Geometry: final body of the model. Coordinates: model frame, mm. Coordinates: 2 decimals unless noted, no trailing zeros. Order: outer loops, then holes, each group sorted by start corner. A loop starts at its lowest first (then second) coordinate and runs counter-clockwise, first axis right, second up. Notation, with made-up numbers: M 26,80 L 58,80 A31 cw 58,115 Z; hole C 88.25,-30 d10. An arc over 180 degrees is marked long. Write item = value, one per line. Start each with the question number.
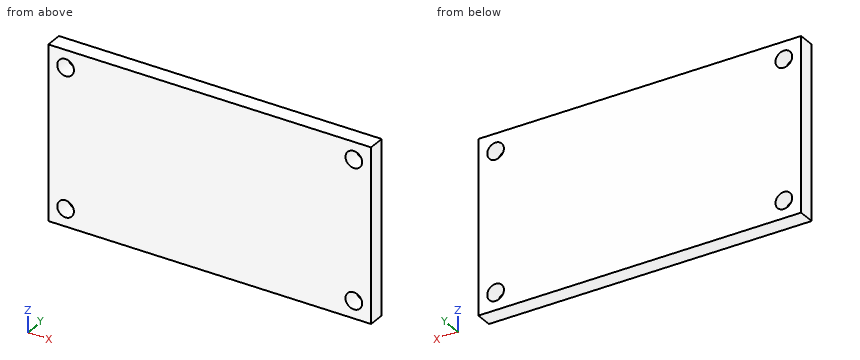
```python
from build123d import *

# Parameters (mm, degrees)
SKETCH1_W               = 58
SKETCH1_H               = 31
BOSS_EXTRUDE1_DEPTH     = 3
SKETCH2_R               = 1.5
CUT_EXTRUDE1_DEPTH      = 34.018933962
MIRROR2_COPY_1_SKETCH_R = 1.5
MIRROR2_COPY_1_DEPTH    = 34.018933962


with BuildPart() as part:
    # Sketch1 → Boss-Extrude1 (new body)
    with BuildSketch(Plane(origin=(0, 0, 0), x_dir=(1, 0, 0), z_dir=(0, 1, 0))):
        Rectangle(SKETCH1_W, SKETCH1_H)
    extrude(amount=BOSS_EXTRUDE1_DEPTH)

    # Sketch2 → Cut-Extrude1 (cut, through all)
    with BuildSketch(Plane(origin=(0, 3, 0), x_dir=(1, 0, 0), z_dir=(0, 1, 0))):
        with Locations(Location((-25.9, 12.4, 0), (0, 0, 270))):
            Circle(SKETCH2_R)
    cut_extrude1 = extrude(amount=-CUT_EXTRUDE1_DEPTH, mode=Mode.SUBTRACT)

    # Mirror1: Cut-Extrude1 across plane
    add(cut_extrude1.mirror(Plane.XY), mode=Mode.SUBTRACT)

    # Mirror2: Cut-Extrude1 across plane
    add(cut_extrude1.mirror(Plane(origin=(0, 0, 0), x_dir=(0, 0, 1), z_dir=(1, 0, 0))), mode=Mode.SUBTRACT)

    # Mirror2 copy 1 sketch → Mirror2 copy 1 (cut, through all)
    with BuildSketch(Plane(origin=(0, 3, 0), x_dir=(-1, 0, 0), z_dir=(0, 1, 0))):
        with Locations(Location((-25.9, 12.4, 0), (0, 0, 270))):
            Circle(MIRROR2_COPY_1_SKETCH_R)
    extrude(amount=-MIRROR2_COPY_1_DEPTH, mode=Mode.SUBTRACT)


solid = part.part
```
Item 1: Section query B-B on z = -12.4. Output: boundary loops of the cut face in (x, y), and give its area (3 significant figures).
Item 2: Section query A-A on x = -25. Output: boundary loops of the cut face in (y, z).
Item 3: Material intervals for probe 1 along X at (y, z) = (1.25, 12.4); probe 2 along Z at (x, y) = (25.9, 1.6); probe 3 along X at (y, z) = (0.3, -12), sorted ascending. Write a range as [from, to].
Item 4: Section query C-C on y = 0.85. Output: boundary loops of the cut face in (x, z), and give its area (3 significant figures).
Ans:
q1.outline = M -29,0 L -27.4,0 L -27.4,3 L -29,3 Z; M -24.4,0 L 24.4,0 L 24.4,3 L -24.4,3 Z; M 27.4,0 L 29,0 L 29,3 L 27.4,3 Z
q1.area = 156 mm^2
q2.outline = M 0,-15.5 L 3,-15.5 L 3,-13.6 L 0,-13.6 Z; M 0,-11.2 L 3,-11.2 L 3,11.2 L 0,11.2 Z; M 0,13.6 L 3,13.6 L 3,15.5 L 0,15.5 Z
q3.probe_1 = [-29, -27.4], [-24.4, 24.4], [27.4, 29]
q3.probe_2 = [-15.5, -13.9], [-10.9, 10.9], [13.9, 15.5]
q3.probe_3 = [-29, -27.35], [-24.45, 24.45], [27.35, 29]
q4.outline = M -29,-15.5 L 29,-15.5 L 29,15.5 L -29,15.5 Z; hole C -25.9,-12.4 d3; hole C -25.9,12.4 d3; hole C 25.9,-12.4 d3; hole C 25.9,12.4 d3
q4.area = 1,770 mm^2
